Can you work these out from the model? Positions are in its coordinate system, mm. Round coordinates to 2 decimals unless told otherwise and drop trailing zeros. Order: outer loops, then holes, each group sorted by start corner. A loop starts at its lowest first (then second) coordinate and runs counter-clockwise, first axis right, second up. Notation, with made-up numbers: M 36,-29.75 L 92,-29.75 A15 ccw 92,-24.75 Z; hole C 20.25,37.25 d7. An arc over 180 degrees is marked long. Answer as a JSON object with one key per item and string values. Group by question number.
```python
from build123d import *

# Parameters (mm, degrees)
SKETCH1_W           = 350
SKETCH1_H           = 300
BOSS_EXTRUDE1_DEPTH = 20
SKETCH2_R           = 5
CUT_EXTRUDE1_DEPTH  = 21
SKETCH3_R           = 2.75
CUT_EXTRUDE2_DEPTH  = 20
SKETCH4_R           = 5
CUT_EXTRUDE3_DEPTH  = 20
SKETCH5_R           = 2.75
CUT_EXTRUDE4_DEPTH  = 20
SKETCH6_R           = 16
CUT_EXTRUDE5_DEPTH  = 20
SKETCH7_R           = 2.75
CUT_EXTRUDE6_DEPTH  = 20
SKETCH8_R           = 1
CUT_EXTRUDE7_DEPTH  = 15


with BuildPart() as part:
    # Sketch1 → Boss-Extrude1 (new body)
    with BuildSketch(Plane(origin=(0, 0, 0), x_dir=(1, 0, 0), z_dir=(0, 1, 0))):
        Rectangle(SKETCH1_W, SKETCH1_H)
    extrude(amount=BOSS_EXTRUDE1_DEPTH)

    # Sketch2 → Cut-Extrude1 (cut, through all)
    with BuildSketch(Plane(origin=(0, 20, 0), x_dir=(1, 0, 0), z_dir=(0, 1, 0))):
        with Locations((-150, -125)):
            Circle(SKETCH2_R)
        with Locations((-150, 125)):
            Circle(SKETCH2_R)
        with Locations((150, 125)):
            Circle(SKETCH2_R)
        with Locations((150, -125)):
            Circle(SKETCH2_R)
    extrude(amount=-CUT_EXTRUDE1_DEPTH, mode=Mode.SUBTRACT)

    # Sketch3 → Cut-Extrude2 (cut)
    with BuildSketch(Plane(origin=(0, 20, 0), x_dir=(1, 0, 0), z_dir=(0, 1, 0))):
        with Locations((75, 0)):
            Circle(SKETCH3_R)
        with Locations((99, 0)):
            Circle(SKETCH3_R)
    extrude(amount=-CUT_EXTRUDE2_DEPTH, mode=Mode.SUBTRACT)

    # Sketch4 → Cut-Extrude3 (cut)
    with BuildSketch(Plane(origin=(0, 20, 0), x_dir=(1, 0, 0), z_dir=(0, 1, 0))):
        with Locations((150.5, 0)):
            Circle(SKETCH4_R)
    extrude(amount=-CUT_EXTRUDE3_DEPTH, mode=Mode.SUBTRACT)

    # Sketch5 → Cut-Extrude4 (cut)
    with BuildSketch(Plane(origin=(0, 20, 0), x_dir=(1, 0, 0), z_dir=(0, 1, 0))):
        with Locations((-40, 40)):
            Circle(SKETCH5_R)
        with Locations((40, 40)):
            Circle(SKETCH5_R)
        with Locations((40, -40)):
            Circle(SKETCH5_R)
        with Locations((-40, -40)):
            Circle(SKETCH5_R)
    extrude(amount=-CUT_EXTRUDE4_DEPTH, mode=Mode.SUBTRACT)

    # Sketch6 → Cut-Extrude5 (cut)
    with BuildSketch(Plane(origin=(0, 20, 0), x_dir=(1, 0, 0), z_dir=(0, 1, 0))):
        Circle(SKETCH6_R)
    extrude(amount=-CUT_EXTRUDE5_DEPTH, mode=Mode.SUBTRACT)

    # Sketch7 → Cut-Extrude6 (cut)
    with BuildSketch(Plane(origin=(0, 20, 0), x_dir=(1, 0, 0), z_dir=(0, 1, 0))):
        with Locations((-25, 25)):
            Circle(SKETCH7_R)
        with Locations((25, 25)):
            Circle(SKETCH7_R)
        with Locations((25, -25)):
            Circle(SKETCH7_R)
        with Locations((-25, -25)):
            Circle(SKETCH7_R)
    extrude(amount=-CUT_EXTRUDE6_DEPTH, mode=Mode.SUBTRACT)

    # Sketch8 → Cut-Extrude7 (cut)
    with BuildSketch(Plane(origin=(175, 0, 0), x_dir=(0, 0, -1), z_dir=(1, 0, 0))):
        with Locations((-100, 10)):
            Circle(SKETCH8_R)
        with Locations((100, 10)):
            Circle(SKETCH8_R)
    extrude(amount=-CUT_EXTRUDE7_DEPTH, mode=Mode.SUBTRACT)


solid = part.part
```
1) We'd pull the mould along X, two halves only. Please class faces 1 (the face through (145, 10, 125)), 2 (the face through (-175, 10, 2)), 3 (the face through (-2, 0, -35)): +X half, -X half, draft (parallel to the pull), parting line (faces both ways), or undercut.
2) If we section it at A-A on z = 125: Write out the boundary of the cut face in (x, y), plus the area to 3 significant figures.
3) For pin 1 (1.6 mm diameter, centred on y = 10, z = 100, fed in from +X), with a flat end and sliding along its axis, tell me the tip position at first contact or that it passes through.
4) I need wall thicknesses on line 1 along Z through (x, y) = (-150, 9.5); line 2 along X through (y, z) = (6, 0); line 3 along Z through (x, y) = (25, 5.5). Which ranges of each line are inside material? Lowest first, please.
Findings:
{
 "1": {"face 1": "undercut", "face 2": "-X half", "face 3": "draft"},
 "2": {"outline": "M -175,0 L -155,0 L -155,20 L -175,20 Z; M -145,0 L 145,0 L 145,20 L -145,20 Z; M 155,0 L 175,0 L 175,20 L 155,20 Z", "area": "6,600 mm^2"},
 "3": {"pin 1": "stops at x = 160"},
 "4": {"line 1": "z = -150 to -130, -120 to 120, 130 to 150", "line 2": "x = -175 to -16, 16 to 72.25, 77.75 to 96.25, 101.75 to 145.5, 155.5 to 175", "line 3": "z = -150 to -27.75, -22.25 to 22.25, 27.75 to 150"}
}
